The model under review builds one solid part; all positions refer to its coordinate system, in mm. A direction names the side the tool comes from. Coordinates: 2 decimals unless noted, no trailing zeros. Loops run counter-clockwise (first coordinate to the right, second up) from the corner with the lowest first, then second, coordinate; pieces in that order, holes last. Notation, with made-up numbers: M 73,-36 L 82,-36 A28 ccw 82,-2 Z; hole C -37.75,60 d11. An arc over 180 degrees is marked long. Return JSON: item names as keys, results as strings.
```python
from build123d import *

# Parameters (mm, degrees)
F0_W     = 2.5
F0_H     = 22.25
F0_R     = 4.5
F0_W_2   = 22.5
F0_H_2   = 2.5
F1_DEPTH = 2
F2_DEPTH = 2.5
F3_W     = 2.5
F3_H     = 22.5
F3_R     = 4.5
F3_H_2   = 2.5
F3_W_2   = 22.5
F4_DEPTH = 2
F5_R     = 5
F6_R     = 1


with BuildPart() as f1:
    # F0 (on Top) → F1 (new body)
    with BuildSketch(Plane.XY):
        Polygon((-0.25, -0.25), (-0.25, 0), (-2.75, 0), (-2.75, -2.75), (-0.25, -2.75), align=None)
        with Locations((-1.5, 11.125)):
            Rectangle(F0_W, F0_H)
        with BuildLine():
            Line((-0.25, 22.25), (-0.25, 0))
            Line((-0.25, 0), (-0.25, -0.25))
            Line((-0.25, -0.25), (22.25, -0.25))
            Line((22.25, -0.25), (22.25, 0))
            ThreePointArc((22.25, 0), (15.7331258814, 15.7331258814), (0, 22.25))
            Line((0, 22.25), (-0.25, 22.25))
        make_face()
        with Locations((8.5, 8.5)):
            Circle(F0_R, mode=Mode.SUBTRACT)
        with Locations((11, -1.5)):
            Rectangle(F0_W_2, F0_H_2)
    extrude(amount=-F1_DEPTH)

    # F0 (on Top) → F2 (join)
    with BuildSketch(Plane.XY):
        with Locations((-1.5, 11.125)):
            Rectangle(F0_W, F0_H)
        Polygon((-0.25, -0.25), (-0.25, 0), (-2.75, 0), (-2.75, -2.75), (-0.25, -2.75), align=None)
        with Locations((11, -1.5)):
            Rectangle(F0_W_2, F0_H_2)
    extrude(amount=F2_DEPTH)

    # F3 (on face) → F4 (join)
    with BuildSketch(Plane.XY.offset(2.5)):
        with Locations((-1.5, 11)):
            Rectangle(F3_W, F3_H)
        with BuildLine():
            Line((0, 22.25), (-0.25, 22.25))
            Line((-0.25, 22.25), (-0.25, -0.25))
            Line((-0.25, -0.25), (22.25, -0.25))
            Line((22.25, -0.25), (22.25, 0))
            ThreePointArc((22.25, 0), (15.7331258814, 15.7331258814), (0, 22.25))
        make_face()
        with Locations((8.5, 8.5)):
            Circle(F3_R, mode=Mode.SUBTRACT)
        with Locations((-1.5, -1.5)):
            Rectangle(F3_W, F3_H_2)
        with Locations((11, -1.5)):
            Rectangle(F3_W_2, F3_H_2)
    extrude(amount=F4_DEPTH)

    # F5
    f5_edges = [f1.edges().sort_by_distance(p)[0] for p in [
        (-2.75, -2.75, 1.25),
    ]]
    fillet(f5_edges, radius=F5_R)

    # F6
    f6_edges = [f1.edges().sort_by_distance(p)[0] for p in [
        (12.25, -2.75, 4.5),
        (12.25, -2.75, -2),
        (-1.285534, -1.285534, -2),
    ]]
    fillet(f6_edges, radius=F6_R)


solid = f1.part
```
1. Machinability: for faces 4 (the face through (-2.75, 12, 1)), 5 (the face through (8, 14, 2.5)), which of the approach directions +Z, -Z, +X, -X, +Y, -Y give a long, thin tool a straight path to every point of the face, cutting with its end or side? Answer none if there is none.
Check values:
{"face 4": "+Z, -Z, -X, +Y, -Y", "face 5": "+X, +Y"}
2. Add section D-D on y = 15.25. Give the boundary of the cut face in (x, z), plus the area to 3 significant figures.
Check values:
{"outline": "M -2.75,-1 A1 ccw -1.75,-2 L 16.2,-2 L 16.2,0 L -0.25,0 L -0.25,2.5 L 16.2,2.5 L 16.2,4.5 L -1.75,4.5 A1 ccw -2.75,3.5 Z", "area": "81.6 mm²"}
3. Add section A-A on y = 8.5. Give the boundary of the cut face in (x, z), plus the area to 3 significant figures.
Check values:
{"outline": "M -2.75,-1 A1 ccw -1.75,-2 L 4,-2 L 4,0 L -0.25,0 L -0.25,2.5 L 4,2.5 L 4,4.5 L -1.75,4.5 A1 ccw -2.75,3.5 Z; M 13,-2 L 20.56,-2 L 20.56,0 L 13,0 Z; M 13,2.5 L 20.56,2.5 L 20.56,4.5 L 13,4.5 Z", "area": "63.1 mm²"}
4. Insertion check: pin 1 Ø7 at (x, y) = (8.5, 8.5) entering from -Z (3 decimals); pin 2 Ø2 at (x, z) = (16.5, 0) entering from +Y; pin 3 Ø2 at (x, z) = (15, 2) entering from +Y; pin 4 Ø3 at (x, z) = (8, 1.5) entering from +Y. Each pin has a flat end and moves straight along its axis. Give the tip position at first contact, or say it passes through.
Check values:
{"pin 1": "through", "pin 2": "y = 15.96", "pin 3": "y = 17.18", "pin 4": "y = 21.16"}
5. The part is to be moulded in two halves that separate along Z. For faces 1 (the face through (-2.449, 12.11, -1.715)), 2 (the face through (12.792, 9.852, 3.486)), 3 (the face through (8, 14, 0)), say which applies: released by +Z, released by -Z, zero draft, split by the parting line, or undercut.
Check values:
{"face 1": "released by -Z", "face 2": "zero draft", "face 3": "undercut"}
6. Add section C-C on z = 1.75. Give the boundary of the cut face in (x, y), plus the area to 3 significant figures.
Check values:
{"outline": "M -2.75,2.25 A5 ccw 2.25,-2.75 L 22.25,-2.75 L 22.25,-0.25 L -0.25,-0.25 L -0.25,22.25 L -2.75,22.25 Z", "area": "113 mm²"}
7. Add section B-B on x = 9.75. Give the boundary of the cut face in (y, z).
Check values:
{"outline": "M -2.75,-1 A1 ccw -1.75,-2 L 4.18,-2 L 4.18,0 L -0.25,0 L -0.25,2.5 L 4.18,2.5 L 4.18,4.5 L -1.75,4.5 A1 ccw -2.75,3.5 Z; M 12.82,-2 L 20,-2 L 20,0 L 12.82,0 Z; M 12.82,2.5 L 20,2.5 L 20,4.5 L 12.82,4.5 Z"}
8. To check wall thickness, follow line 1 (Z direction, x = 14.75, y = 5.25); line 2 (Y direction, x = 8.5, z = -0.9); line 3 (Y direction, x = 7.25, z = 2.75). State the ranges of each line that lie inside material, in increasing order.
Check values:
{"line 1": "-2 to 0, 2.5 to 4.5", "line 2": "-2.75 to 4, 13 to 20.56", "line 3": "-2.75 to 4.18, 12.82 to 21.04"}
